Here's how the part is built. I have some questions about the finished solid (model axes, mm). Give positions to 0.01 mm unless a question says otherwise; leave off trailing zeros. Write each loop counter-clockwise with the first axis right and the second up, starting at its lowest first coordinate (ties: lowest second). Pieces come first, ordered by that corner, then holes. Notation, with made-up numbers: (77, -37) - (86, -37) arc R19 cw to (86, -8) - close; hole circle Ø9 at (-24, -11.75). An arc over 180 degrees is marked (long way). Use one line per item in the form item = value. Start each with the question number.
from build123d import *

# Parameters (mm, degrees)
SKETCH1_W                 = 76.2
SKETCH1_H                 = 63.5
BOSS_EXTRUDE1_DEPTH       = 1.5
FILLET1_R                 = 3.175
F_4_CLEARANCE_HOLE1_D     = 3.2639
F_4_CLEARANCE_HOLE1_DEPTH = 6.619425513
F_4_CLEARANCE_HOLE1_TIP   = 0.980574487


with BuildPart() as part:
    # Sketch1 → Boss-Extrude1 (new body, symmetric)
    with BuildSketch(Plane(origin=(0, 0, 0), x_dir=(1, 0, 0), z_dir=(0, 1, 0))):
        Rectangle(SKETCH1_W, SKETCH1_H)
    extrude(amount=BOSS_EXTRUDE1_DEPTH, both=True)

    # Fillet1
    fillet1_edges = [part.edges().sort_by_distance(p)[0] for p in [
        (38.1, 0, 31.75),
        (-38.1, 0, 31.75),
        (-38.1, 0, -31.75),
        (38.1, 0, -31.75),
    ]]
    fillet(fillet1_edges, radius=FILLET1_R)

    # #4 Clearance Hole1
    with Locations(Plane(origin=(0, 1.5, 0), x_dir=(1, 0, 0), z_dir=(0, 1, 0))):
        with Locations((-34.125, 0), (-30.315, -23.045), (0, -26.77), (30.315, -23.045), (34.125, 0), (30.315, 23.045), (0, 26.77), (-30.315, 23.045)):
            Hole(F_4_CLEARANCE_HOLE1_D / 2, depth=F_4_CLEARANCE_HOLE1_DEPTH)
            with Locations((0, 0, -(F_4_CLEARANCE_HOLE1_DEPTH + F_4_CLEARANCE_HOLE1_TIP / 2))):  # 118° drill point
                Cone(0, F_4_CLEARANCE_HOLE1_D / 2, F_4_CLEARANCE_HOLE1_TIP, mode=Mode.SUBTRACT)


solid = part.part
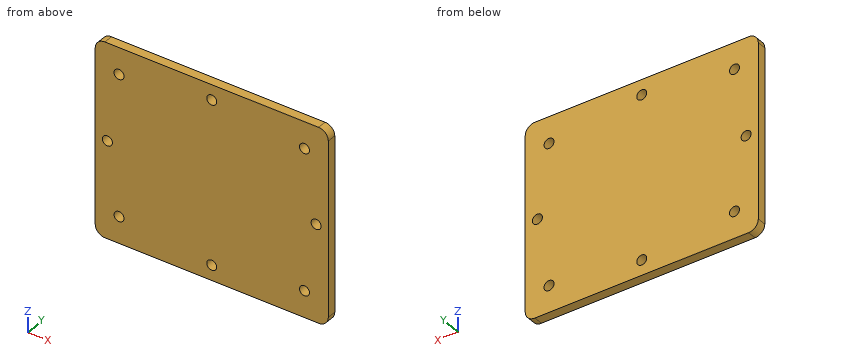
1. I want a section at A-A, the plane z = 0. List the corners of the cut face in (x, y) for me, then the cut area to 3 significant figures.
2. I want a section at C-C, the plane y = 0.4. Give the number of separate pieces and of enclosed holes in the cut face, then the cut area to 3 significant figures.
3. Please list where these lines run through material, in increasing order: line 1 (Z direction, x = 0, y = 0.2); line 2 (X direction, y = -0.1, z = -26.77); line 3 (Z direction, x = 30, y = -0.5).
4. I want a section at B-B, the plane z = -26.77. List the corners of the cut face in (x, y) for me, then the cut area to 3 significant figures.
5. For P1, Ø4, axis at x = 30.315, z = -23.045, coming from the +Y side, with a flat end and sliding along its axis, tell me the tip position at first contact or that it passes through.
Result sheet:
q1.outline = (-38.1, -1.5) - (-35.76, -1.5) - (-35.76, 1.5) - (-38.1, 1.5) - close; (-32.49, -1.5) - (32.49, -1.5) - (32.49, 1.5) - (-32.49, 1.5) - close; (35.76, -1.5) - (38.1, -1.5) - (38.1, 1.5) - (35.76, 1.5) - close
q1.area = 209 mm2
q2.separate_pieces = 1
q2.enclosed_holes = 8
q2.area = 4,760 mm2
q3.line_1 = -31.75 to -28.4, -25.14 to 25.14, 28.4 to 31.75
q3.line_2 = -38.1 to -1.63, 1.63 to 38.1
q3.line_3 = -31.75 to -24.65, -21.44 to 21.44, 24.65 to 31.75
q4.outline = (-38.1, -1.5) - (-1.63, -1.5) - (-1.63, 1.5) - (-38.1, 1.5) - close; (1.63, -1.5) - (38.1, -1.5) - (38.1, 1.5) - (1.63, 1.5) - close
q4.area = 219 mm2
q5.P1 = 1.5
